```python
from build123d import *

# Parameters (mm, degrees)
SKETCH1_W                       = 63.5
SKETCH1_H                       = 24.13
BOSS_EXTRUDE1_DEPTH             = 4.064
BOSS_EXTRUDE2_REACH             = 36.207
BOSS_EXTRUDE2_DIRECTION_2_REACH = 36.207
CUT_EXTRUDE1_DEPTH              = 4.064
CUT_EXTRUDE1_DEPTH_BACK         = 66.752974943
SKETCH4_R                       = 8.636
FILLET1_R                       = 2.54
CUT_EXTRUDE2_DEPTH              = 73.348315655
BOSS_EXTRUDE3_DEPTH             = 2.54
BOSS_EXTRUDE4_START             = 2.54
BOSS_EXTRUDE4_DEPTH             = 2.54
BOSS_EXTRUDE5_DEPTH             = 3.81
CUT_EXTRUDE3_DEPTH              = 64.061052508
BOSS_EXTRUDE6_START             = -23.114
SKETCH12_W                      = 44.831
SKETCH12_H                      = 27.027043781
BOSS_EXTRUDE6_DEPTH             = 23.114
BOSS_EXTRUDE7_DEPTH             = 7.874
CUT_EXTRUDE4_START              = -6.219751
CUT_EXTRUDE4_DEPTH              = 6.219751
CUT_EXTRUDE5_DEPTH              = 27.027043781
SKETCH17_W                      = 6.9977
SKETCH17_H                      = 3.556
BOSS_EXTRUDE8_DEPTH             = 13.97
SKETCH18_W                      = 6.389869694
SKETCH18_H                      = 3.556
BOSS_EXTRUDE9_DEPTH             = 13.97
SKETCH19_W                      = 31.75
SKETCH19_H                      = 7.112
CUT_EXTRUDE6_DEPTH              = 13.97
CUT_EXTRUDE7_REACH              = 87.043
SKETCH20_R                      = 1.7145
FILLET2_R                       = 2.54
FILLET3_R                       = 2.54
FILLET4_R                       = 2.54
BOSS_EXTRUDE10_DEPTH            = 29.21
BOSS_EXTRUDE11_DEPTH            = 27.027043781
BOSS_EXTRUDE16_DEPTH            = 6.35
FILLET5_R                       = 6.35
FILLET6_R                       = 3.81


with BuildPart() as part:
    # Sketch1 → Boss-Extrude1 (new body)
    with BuildSketch(Plane(origin=(0, 0, 0), x_dir=(1, 0, 0), z_dir=(0, 1, 0))):
        Rectangle(SKETCH1_W, SKETCH1_H)
    extrude(amount=BOSS_EXTRUDE1_DEPTH)

    # Boss-Extrude2: up to this face of the body (flat: up to its plane)
    boss_extrude2_end = Plane(part.part.faces().sort_by_distance((0, 2.032, 12.065))[0])
    # Sketch2 → Boss-Extrude2 (add, up to the picked face)
    with BuildSketch(Plane.XY, mode=Mode.PRIVATE) as boss_extrude2_sk1:
        with BuildLine():
            Line((0, 4.064), (-26.716755185, 4.064))
            Line((-26.716755185, 4.064), (-31.571041118, 27.367716778))
            ThreePointArc((-31.571041118, 27.367716778), (-27.221246487, 47.076161415), (-11.87173913, 60.180974548))
            ThreePointArc((-11.87173913, 60.180974548), (-8.566242036, 58.774955714), (-9.97226087, 55.46945862))
            ThreePointArc((-9.97226087, 55.46945862), (-26.181898149, 25.654914521), (0, 4.064))
        make_face()
    boss_extrude2_tool1 = split(extrude(boss_extrude2_sk1.sketch, amount=BOSS_EXTRUDE2_REACH, mode=Mode.PRIVATE), bisect_by=boss_extrude2_end, keep=Keep.BOTH, mode=Mode.PRIVATE)
    add(boss_extrude2_tool1.solids().sort_by(Axis((-9.165723, 58.533271, 0), (0, 0, 1)))[0])

    # Boss-Extrude2 direction 2: up to this face of the body (flat: up to its plane)
    boss_extrude2_direction_2_end = Plane(part.part.faces().sort_by_distance((0, 2.032, -12.065))[0])
    # Sketch2 → Boss-Extrude2 direction 2 (add, up to the picked face)
    with BuildSketch(Plane.XY, mode=Mode.PRIVATE) as boss_extrude2_direction_2_sk1:
        with BuildLine():
            Line((0, 4.064), (-26.716755185, 4.064))
            Line((-26.716755185, 4.064), (-31.571041118, 27.367716778))
            ThreePointArc((-31.571041118, 27.367716778), (-27.221246487, 47.076161415), (-11.87173913, 60.180974548))
            ThreePointArc((-11.87173913, 60.180974548), (-8.566242036, 58.774955714), (-9.97226087, 55.46945862))
            ThreePointArc((-9.97226087, 55.46945862), (-26.181898149, 25.654914521), (0, 4.064))
        make_face()
    boss_extrude2_direction_2_tool1 = split(extrude(boss_extrude2_direction_2_sk1.sketch, amount=-BOSS_EXTRUDE2_DIRECTION_2_REACH, mode=Mode.PRIVATE), bisect_by=boss_extrude2_direction_2_end, keep=Keep.BOTH, mode=Mode.PRIVATE)
    add(boss_extrude2_direction_2_tool1.solids().sort_by(Axis((-9.165723, 58.533271, 0), (0, 0, -1)))[0])

    # Sketch4 → Cut-Extrude1 (cut, two sides: drawn at the far end of the back side and taken through both)
    with BuildSketch(Plane(origin=(0, 4.064, 0), x_dir=(1, 0, 0), z_dir=(0, 1, 0)).offset(-CUT_EXTRUDE1_DEPTH_BACK)):
        with Locations(Location((0, 0, 0), (0, 0, 270))):
            Circle(SKETCH4_R)
    extrude(amount=CUT_EXTRUDE1_DEPTH + CUT_EXTRUDE1_DEPTH_BACK, mode=Mode.SUBTRACT)

    # Fillet1
    fillet1_edges = [part.edges().sort_by_distance(p)[0] for p in [
        (-8.636, 5.50091846, 0),
        (8.636, 4.064, 0),
    ]]
    fillet(fillet1_edges, radius=FILLET1_R)

    # Sketch6 → Cut-Extrude2 (cut, through all)
    with BuildSketch(Plane.XY.offset(12.065)):
        Polygon((-31.75, 4.064), (-26.716755185, 4.064), (-25.870202757, 0), (-31.75, 0), align=None)
    extrude(amount=-CUT_EXTRUDE2_DEPTH, mode=Mode.SUBTRACT)

    # Sketch8 → Boss-Extrude3 (add)
    with BuildSketch(Plane.XY.offset(12.065)):
        with BuildLine():
            Line((31.75, 0), (31.75, 7.874))
            Line((31.75, 7.874), (-4.274632474, 7.874))
            ThreePointArc((-4.274632474, 7.874), (-23.508790492, 29.710248048), (-9.97226087, 55.46945862))
            ThreePointArc((-9.97226087, 55.46945862), (-8.566242036, 58.774955714), (-11.87173913, 60.180974548))
            ThreePointArc((-11.87173913, 60.180974548), (-27.221246487, 47.076161415), (-31.571041118, 27.367716778))
            Line((-31.571041118, 27.367716778), (-25.870202757, 0))
            Line((-25.870202757, 0), (31.75, 0))
        make_face()
    extrude(amount=BOSS_EXTRUDE3_DEPTH)

    # Sketch9 → Boss-Extrude4 (add)
    with BuildSketch(Plane(origin=(0, 0, -12.065), x_dir=(-1, 0, 0), z_dir=(0, 0, -1)).offset(BOSS_EXTRUDE4_START)):
        with BuildLine():
            Line((-31.75, 0), (-31.75, 7.874))
            Line((-31.75, 7.874), (4.274632474, 7.874))
            ThreePointArc((4.274632474, 7.874), (23.508790492, 29.710248048), (9.97226087, 55.46945862))
            ThreePointArc((9.97226087, 55.46945862), (8.566242036, 58.774955714), (11.87173913, 60.180974548))
            ThreePointArc((11.87173913, 60.180974548), (27.221246487, 47.076161415), (31.571041118, 27.367716778))
            Line((31.571041118, 27.367716778), (25.870202757, 0))
            Line((25.870202757, 0), (-31.75, 0))
        make_face()
    extrude(amount=-BOSS_EXTRUDE4_DEPTH)

    # Sketch10 → Boss-Extrude5 (add)
    with BuildSketch(Plane(origin=(0, 4.064, 0), x_dir=(1, 0, 0), z_dir=(0, 1, 0))):
        with BuildLine():
            Line((10.218295125, 14.605), (10.218295125, 12.065))
            ThreePointArc((10.218295125, 12.065), (22.283295125, 0), (10.218295125, -12.065))
            Line((10.218295125, -12.065), (10.218295125, -14.605))
            ThreePointArc((10.218295125, -14.605), (24.823295125, 0), (10.218295125, 14.605))
        make_face()
    extrude(amount=BOSS_EXTRUDE5_DEPTH)

    # Sketch11 → Cut-Extrude3 (cut, through all)
    with BuildSketch(Plane(origin=(0, 7.874, 0), x_dir=(1, 0, 0), z_dir=(0, 1, 0))):
        with BuildLine():
            Line((10.218295125, 14.605), (31.75, 14.605))
            Line((31.75, 14.605), (31.75, -14.605))
            Line((31.75, -14.605), (10.218295125, -14.605))
            ThreePointArc((10.218295125, -14.605), (24.823295125, 0), (10.218295125, 14.605))
        make_face()
    extrude(amount=-CUT_EXTRUDE3_DEPTH, mode=Mode.SUBTRACT)

    # Sketch12 → Boss-Extrude6 (add)
    with BuildSketch(Plane.XZ.offset(BOSS_EXTRUDE6_START)):
        with Locations((-8.8011, -28.11852189)):
            Rectangle(SKETCH12_W, SKETCH12_H)
    extrude(amount=BOSS_EXTRUDE6_DEPTH)

    # Sketch13 → Boss-Extrude7 (add)
    with BuildSketch(Plane.XZ):
        Polygon((10.218295125, -14.605), (13.6144, -14.605), (13.6144, -13.335525526), align=None)
    extrude(amount=-BOSS_EXTRUDE7_DEPTH)

    # Sketch14 → Cut-Extrude4 (cut)
    with BuildSketch(Plane.XY.offset(-14.605).offset(CUT_EXTRUDE4_START)):
        with BuildLine():
            Line((0, 13.017313502), (18.620278687, 13.017313502))
            Line((18.620278687, 13.017313502), (17.716686498, 30.734))
            ThreePointArc((17.716686498, 30.734), (-12.527589163, 43.261589163), (0, 13.017313502))
        make_face()
    extrude(amount=CUT_EXTRUDE4_DEPTH, mode=Mode.SUBTRACT)

    # Sketch16 → Cut-Extrude5 (cut)
    with BuildSketch(Plane.XY.offset(-14.605)):
        Polygon((-31.2166, 23.114), (-30.684969694, 23.114), (-25.870202757, 0), (-31.2166, 0), align=None)
    extrude(amount=-CUT_EXTRUDE5_DEPTH, mode=Mode.SUBTRACT)

    # Sketch17 → Boss-Extrude8 (add)
    with BuildSketch(Plane(origin=(0, 23.114, 0), x_dir=(1, 0, 0), z_dir=(0, 1, 0))):
        with Locations((10.11555, 34.413750632)):
            Rectangle(SKETCH17_W, SKETCH17_H)
    extrude(amount=BOSS_EXTRUDE8_DEPTH)

    # Sketch18 → Boss-Extrude9 (add)
    with BuildSketch(Plane(origin=(0, 23.114, 0), x_dir=(1, 0, 0), z_dir=(0, 1, 0))):
        with Locations((-27.490034847, 34.413750632)):
            Rectangle(SKETCH18_W, SKETCH18_H)
    extrude(amount=BOSS_EXTRUDE9_DEPTH)

    # Sketch19 → Cut-Extrude6 (cut)
    with BuildSketch(Plane(origin=(0, 37.084, 0), x_dir=(1, 0, 0), z_dir=(0, 1, 0))):
        with Locations((-8.8392, 36.191750632)):
            Rectangle(SKETCH19_W, SKETCH19_H)
    extrude(amount=-CUT_EXTRUDE6_DEPTH, mode=Mode.SUBTRACT)

    # Sketch20 → Cut-Extrude7 (cut, up to next)
    with BuildSketch(Plane(origin=(0, 0, -36.191750632), x_dir=(-1, 0, 0), z_dir=(0, 0, -1)), mode=Mode.PRIVATE) as cut_extrude7_sk1:
        with Locations((27.75585, 30.734)):
            Circle(SKETCH20_R)
    cut_extrude7_tool1 = extrude(cut_extrude7_sk1.sketch, amount=-CUT_EXTRUDE7_REACH, mode=Mode.PRIVATE) & part.part
    # Sketch20 → Cut-Extrude7 (cut, up to next)
    with BuildSketch(Plane(origin=(0, 0, -36.191750632), x_dir=(-1, 0, 0), z_dir=(0, 0, -1)), mode=Mode.PRIVATE) as cut_extrude7_sk2:
        with Locations((-10.11555, 30.734)):
            Circle(SKETCH20_R)
    cut_extrude7_tool2 = extrude(cut_extrude7_sk2.sketch, amount=-CUT_EXTRUDE7_REACH, mode=Mode.PRIVATE) & part.part
    add(cut_extrude7_tool1.solids().sort_by_distance((-27.75585, 30.734, -36.191751))[0], mode=Mode.SUBTRACT)
    add(cut_extrude7_tool2.solids().sort_by_distance((10.11555, 30.734, -36.191751))[0], mode=Mode.SUBTRACT)

    # Fillet2
    fillet2_edges = [part.edges().sort_by_distance(p)[0] for p in [
        (10.3251, 23.114, -36.191750632),
    ]]
    fillet(fillet2_edges, radius=FILLET2_R)

    # Fillet3
    fillet3_edges = [part.edges().sort_by_distance(p)[0] for p in [
        (-27.699584847, 23.114, -36.191750632),
    ]]
    fillet(fillet3_edges, radius=FILLET3_R)

    # Fillet4
    fillet4_edges = [part.edges().sort_by_distance(p)[0] for p in [
        (13.6144, 37.084, -34.413750632),
        (-30.684969694, 37.084, -34.413750632),
    ]]
    fillet(fillet4_edges, radius=FILLET4_R)

    # Sketch26 → Boss-Extrude10 (add)
    with BuildSketch(Plane.XY.offset(14.605)):
        Polygon((-25.870202757, 0), (-31.653563464, 0), (-31.571041118, 27.367716778), align=None)
    extrude(amount=-BOSS_EXTRUDE10_DEPTH)

    # Sketch22 → Boss-Extrude11 (add)
    with BuildSketch(Plane(origin=(0, 0, -14.605), x_dir=(-1, 0, 0), z_dir=(0, 0, -1))):
        Polygon((30.684969694, 23.114), (31.583867423, 23.114), (31.653563464, 0), (25.870202757, 0), align=None)
    extrude(amount=BOSS_EXTRUDE11_DEPTH)

    # Sketch23 → Boss-Extrude16 (add)
    with BuildSketch(Plane.XZ):
        with BuildLine():
            Line((-15.554631727, 14.605), (-44.353563464, 14.605))
            Line((-44.353563464, 14.605), (-44.353563464, -41.632043781))
            ThreePointArc((-44.353563464, -41.632043781), (-40.609144413, -50.636907459), (-31.583867423, -54.331852538))
            Line((-31.583867423, -54.331852538), (13.6144, -54.332043781))
            Line((13.6144, -54.332043781), (13.6144, -35.10352189))
            Line((13.6144, -35.10352189), (-15.554631727, -35.10352189))
            Line((-15.554631727, -35.10352189), (-15.554631727, 14.605))
        make_face()
        with BuildLine():
            Line((-34.701563464, 8.07647811), (-34.701563464, -35.10352189))
            ThreePointArc((-34.701563464, -35.10352189), (-38.003563464, -38.40552189), (-41.305563464, -35.10352189))
            Line((-41.305563464, -35.10352189), (-41.305563464, 8.07647811))
            ThreePointArc((-41.305563464, 8.07647811), (-38.003563464, 11.37847811), (-34.701563464, 8.07647811))
        make_face(mode=Mode.SUBTRACT)
        with BuildLine():
            Line((-24.859733712, -44.680043781), (6.890266288, -44.680043781))
            ThreePointArc((6.890266288, -44.680043781), (10.192266288, -47.982043781), (6.890266288, -51.284043781))
            Line((6.890266288, -51.284043781), (-24.859733712, -51.284043781))
            ThreePointArc((-24.859733712, -51.284043781), (-28.161733712, -47.982043781), (-24.859733712, -44.680043781))
        make_face(mode=Mode.SUBTRACT)
    extrude(amount=-BOSS_EXTRUDE16_DEPTH)

    # Fillet5
    fillet5_edges = [part.edges().sort_by_distance(p)[0] for p in [
        (13.6144, 3.175, -54.332043781),
        (-44.353563464, 3.175, 14.605),
    ]]
    fillet(fillet5_edges, radius=FILLET5_R)

    # Fillet6
    fillet6_edges = [part.edges().sort_by_distance(p)[0] for p in [
        (-31.609141812, 14.732, -41.632043781),
    ]]
    fillet(fillet6_edges, radius=FILLET6_R)


solid = part.part
```
Geometry: final body of the model. Coordinates: model frame, mm. A direction names the side the tool comes from. Round coordinates to 2 decimals unless told otherwise and drop trailing zeros. Order: outer loops, then holes, each group sorted by start corner. A loop starts at its lowest first (then second) coordinate and runs counter-clockwise, first axis right, second up. Notation, with made-up numbers: (-8, 14.25) -> (3, 14.25) arc R24 ccw to (3, 36.25) -> close; hole circle Ø6 at (40, 31). An arc over 180 degrees is marked (long way). Use one line per item in the form item = value.
(1) Section C-C on x = 20. Return loops of the section in (y, z).
Results list:
outline = (0, -10.85) -> (7.87, -10.85) -> (7.87, -7.06) -> (4.06, -7.06) -> (4.06, 7.06) -> (7.87, 7.06) -> (7.87, 10.85) -> (0, 10.85) -> close
(2) Section D-D on z = 0. Count the separate pieces of the cut face and the enclosed holes in it, and give its area (3 significant figures).
Results list:
separate_pieces = 3
enclosed_holes = 0
area = 673 mm^2
(3) Section B-B on x = -18.5. Return loops of the section in (y, z) (3 decimals), and give its area (3 significant figures).
Results list:
outline = (0, -54.332) -> (6.35, -54.332) -> (6.35, -51.284) -> (0, -51.284) -> close; (0, -44.68) -> (6.35, -44.68) -> (6.35, -41.632) -> (23.114, -41.632) -> (23.114, -14.605) -> (17.287, -14.605) -> (17.287, -12.065) -> (11.524, -12.065) -> (11.524, 12.065) -> (17.287, 12.065) -> (17.287, 14.605) -> (0, 14.605) -> close; (48.232, -14.605) -> (56.537, -14.605) -> (56.537, 14.605) -> (48.232, 14.605) -> (48.232, 12.065) -> (49.944, 12.065) -> (49.944, -12.065) -> (48.232, -12.065) -> close
area = 1,230 mm^2
(4) First-contact query: pin 1 Ø8 at (x, y) = (-5.5, 16.5) entering from +Z (3 decimals); pin 2 Ø1.7 at (x, z) = (-26.5, -34.5) entering from +Y; pin 3 Ø10 at (y, z) = (44, -14.5) entering from +X; pin 4 Ø8.5 at (x, z) = (3, 2) entering from +Y. Flat tips, straight axial feed; report the tip coordinate or a pass-through.
Results list:
pin_1 = -14.605
pin_2 = 37.08
pin_3 = -17.9
pin_4 = through
(5) Ray query, probe 1 along X at (y, z) = (1.55, 0); probe 2 along Z at (x, y) = (0, 1.1) (3 decimals); probe 3 along Z at (x, y) = (-16.5, 6) (3 decimals). Return the intervals inside material, ascending. Write a range as [from, to].
Results list:
probe_1 = [-44.35, -41.31], [-34.7, -8.64], [8.64, 24.82]
probe_2 = [-54.332, -51.284], [-44.68, -8.636], [8.636, 14.605]
probe_3 = [-54.332, -51.284], [-44.68, 14.605]
(6) Section A-A on y = 24.5. Return loops of the section in (x, z) (3 decimals), and give its area (3 significant figures).
Results list:
outline = (-31.58, -14.605) -> (-22.325, -14.605) -> (-22.325, -12.065) -> (-25.931, -12.065) -> (-25.931, 12.065) -> (-22.325, 12.065) -> (-22.325, 14.605) -> (-31.58, 14.605) -> close; (-30.685, -36.469) -> (-24.714, -36.469) -> (-24.714, -32.636) -> (-30.685, -32.636) -> close; (7.036, -36.469) -> (13.614, -36.469) -> (13.614, -32.636) -> (7.036, -32.636) -> close
area = 231 mm^2
(7) Access query for faces 4 (the face through (-34.702, 3, -13)), 5 (the face through (-30.46, 14.62, -40.55)), 6 (the face through (22.1, 7.874, -3.2)). Directions: +Z, -Z, +X, -X, +Y, -Y. A direction counts if a zero-diameter tool reaches every point of the face in a straight line with its end or side. Return the directions, or none.
Results list:
face_4 = +Y, -Y
face_5 = -Z, -X, +Y
face_6 = +Z, +X, +Y
(8) Draft query along Z for faces 1 (the face through (-24.714, 30, -34)), 2 (the face through (-28, 33, -36.192)), 3 (the face through (13, 4.064, 0)). Return one class per face: pulls with the +Z half, pulls with the -Z half, needs draft (parallel to the pull), parting line crosses it, or undercut.
Results list:
face_1 = needs draft
face_2 = pulls with the -Z half
face_3 = undercut
